from build123d import *

# Parameters (mm, degrees)
EXTRUDE_1_DEPTH     = 25
EXTRUDE_2_DEPTH     = 36
SKETCH_3_W          = 15
SKETCH_3_H          = 6
EXTRUDE_3_DEPTH     = 12
SKETCH_4_R          = 0.95
CUT_EXTRUDE_1_DEPTH = 21
SKETCH_5_R          = 4
SKETCH_5_R_2        = 1.45
EXTRUDE_4_DEPTH     = 20
EXTRUDE_4_2_DEPTH   = 20
SKETCH_6_R          = 1.75
CUT_EXTRUDE_2_DEPTH = 20
SKETCH_7_R          = 2.5
CUT_EXTRUDE_3_DEPTH = 2
CUT_EXTRUDE_4_DEPTH = 52.148040055
FILLET_4_R          = 1
SKETCH_9_W          = 2
SKETCH_9_H          = 14
EXTRUDE_5_DEPTH     = 20


with BuildPart() as part:
    # Sketch 1 → Extrude 1 (new, symmetric)
    with BuildSketch(Plane.XY):
        Polygon((0, 0), (9.650045346, 0), (39.194277936, -5.20944533), (39.888870647, -1.270214318), (10, 4), (0, 4), align=None)
    extrude_1 = extrude(amount=EXTRUDE_1_DEPTH, both=True)

    # Sketch 2 → Extrude 2 (add)
    with BuildSketch(Plane.XY.offset(25)):
        Polygon((22.162331093, 1.85545288), (22.483580221, 3.677347223), (37.255696517, 1.072624558), (36.934447388, -0.749269785), align=None)
    extrude_2 = extrude(amount=-EXTRUDE_2_DEPTH)

    # Sketch 3 → Extrude 3 (add)
    with BuildSketch(Plane(origin=(1.306826311, 7.411380301, 0), x_dir=(0.9848077530122079, -0.1736481776669312, 0), z_dir=(0.1736481776669312, 0.9848077530122079, 0))):
        with Locations((29.003439474, -22)):
            Rectangle(SKETCH_3_W, SKETCH_3_H)
        with Locations((29.003439474, 7.8)):
            Rectangle(SKETCH_3_W, SKETCH_3_H)
    extrude_3 = extrude(amount=EXTRUDE_3_DEPTH)

    # Sketch 4 → Cut-Extrude 1 (cut)
    with BuildSketch(Plane(origin=(35.948870205, -6.338755743, 0), x_dir=(0, 0, -1), z_dir=(0.9848077530122081, -0.17364817766693072, 0))):
        with Locations(Location((-20.95, 14.025712789, 0), (0, 0, 90))):
            Circle(SKETCH_4_R)
        with Locations(Location((6.75, 14.025712789, 0), (0, 0, 90))):
            Circle(SKETCH_4_R)
    cut_extrude_1 = extrude(amount=-CUT_EXTRUDE_1_DEPTH, mode=Mode.SUBTRACT)

    # Mirror 1: Extrude 1, Extrude 2, Extrude 3, Cut-Extrude 1 across plane
    add(extrude_1.mirror(Plane(origin=(0, 0, 0), x_dir=(0, 0, 1), z_dir=(1, 0, 0))))
    add(extrude_2.mirror(Plane(origin=(0, 0, 0), x_dir=(0, 0, 1), z_dir=(1, 0, 0))))
    add(extrude_3.mirror(Plane(origin=(0, 0, 0), x_dir=(0, 0, 1), z_dir=(1, 0, 0))))
    add(cut_extrude_1.mirror(Plane(origin=(0, 0, 0), x_dir=(0, 0, 1), z_dir=(1, 0, 0))), mode=Mode.SUBTRACT)

    # Sketch 6 → Cut-Extrude 2 (cut)
    with BuildSketch(Plane(origin=(0, 4, 0), x_dir=(1, 0, 0), z_dir=(0, 1, 0))):
        with Locations(Location((0, -20, 0), (0, 0, 180))):
            Circle(SKETCH_6_R)
        with Locations((-13, 9.5)):
            Circle(SKETCH_6_R)
        with Locations(Location((13, 9.5, 0), (0, 0, 180))):
            Circle(SKETCH_6_R)
    extrude(amount=-CUT_EXTRUDE_2_DEPTH, mode=Mode.SUBTRACT)

    # Sketch 7 → Cut-Extrude 3 (cut)
    with BuildSketch(Plane(origin=(0, 4, 0), x_dir=(1, 0, 0), z_dir=(0, 1, 0))):
        with Locations(Location((-13, 9.5, 0), (0, 0, 180))):
            Circle(SKETCH_7_R)
        with Locations(Location((13, 9.5, 0), (0, 0, 180))):
            Circle(SKETCH_7_R)
    extrude(amount=-CUT_EXTRUDE_3_DEPTH, mode=Mode.SUBTRACT)

    # Sketch 8 → Cut-Extrude 4 (cut, through all)
    with BuildSketch(Plane(origin=(0, 4, 0), x_dir=(1, 0, 0), z_dir=(0, 1, 0))):
        Polygon((-4, 23), (-1, 23), (-1, 25), (1, 25), (1, 23), (4, 23), (4, 14), (-4, 14), align=None)
    extrude(amount=-CUT_EXTRUDE_4_DEPTH, mode=Mode.SUBTRACT)

    # Fillet 4
    fillet_4_edges = [part.edges().sort_by_distance(p)[0] for p in [
        (4, 2, -23),
        (4, 2, -14),
        (-4, 2, -14),
        (-4, 2, -23),
        (1, 2, -23),
        (-1, 2, -23),
    ]]
    fillet(fillet_4_edges, radius=FILLET_4_R)



with BuildPart() as body_2:
    # Sketch 5 → Extrude 4 (new body)
    with BuildSketch(Plane(origin=(0, 4, 0), x_dir=(1, 0, 0), z_dir=(0, 1, 0))):
        with Locations(Location((0, -12, 0), (0, 0, 180))):
            Circle(SKETCH_5_R)
        with Locations(Location((0, -12, 0), (0, 0, 180))):
            Circle(SKETCH_5_R_2, mode=Mode.SUBTRACT)
    extrude(amount=EXTRUDE_4_DEPTH)


with BuildPart() as body_3:
    # Sketch 5 → Extrude 4 2 (new body)
    with BuildSketch(Plane(origin=(0, 4, 0), x_dir=(1, 0, 0), z_dir=(0, 1, 0))):
        with Locations(Location((0, 8, 0), (0, 0, 180))):
            Circle(SKETCH_5_R)
        with Locations(Location((0, 8, 0), (0, 0, 180))):
            Circle(SKETCH_5_R_2, mode=Mode.SUBTRACT)
    extrude(amount=EXTRUDE_4_2_DEPTH)


with BuildPart() as part_1:
    add(part.part)

    add(body_2.part)  # Extrude 5 merges body 2

    add(body_3.part)  # Extrude 5 merges body 3
    # Sketch 9 → Extrude 5 (add)
    with BuildSketch(Plane(origin=(0, 4, 0), x_dir=(1, 0, 0), z_dir=(0, 1, 0))):
        with Locations((0, -2)):
            Rectangle(SKETCH_9_W, SKETCH_9_H)
    extrude(amount=EXTRUDE_5_DEPTH)


solid = part_1.part
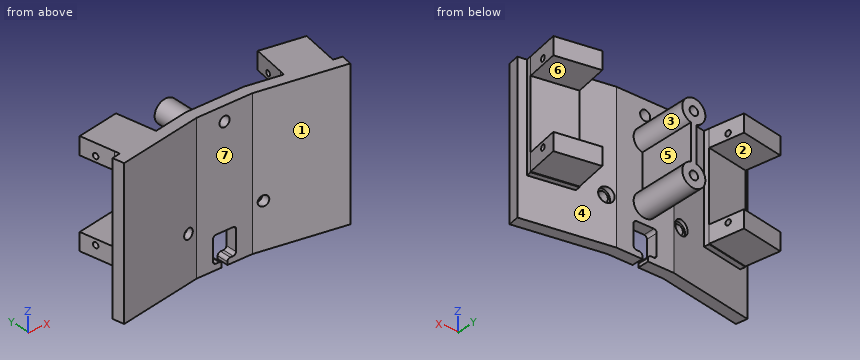
Here's how the part is built. I have some questions about the finished solid (model axes, mm). Face numbers are marked on the shaded views. A direction names the side the tool comes from. Round coordinates to 2 decimals unless told otherwise and drop trailing zeros. Order: outer loops, then holes, each group sorted by start corner. A loop starts at its lowest first (then second) coordinate and runs counter-clockwise, first axis right, second up. Notation, with made-up numbers: M 27.5,78.25 L 53.5,78.25 A36 cw 53.5,112.25 Z; hole C 47,48.5 d1. An arc over 180 degrees is marked long. Return JSON: item names as keys, results as strings. Group by question number.
1. If we section it at A-A on x = 0: List the corners of the cut face in (y, z) for me, then the cut area to 3 significant figures.
2. If we section it at D-D on x = -13: List the corners of the cut face in (y, z) for me, then the cut area to 3 significant figures.
3. If we section it at B-B on z = 12: List the corners of the cut face in (x, y) for me.
4. If we mould it in two halves opening along X, with no side actions, what happens to the marked faces 4, 5, 6 and 7? For each: pulls with the +X half, pulls with the -X half, needs draft (parallel to the pull), parting line crosses it, or undercut.
5. On a 3-axis mill with a long thin cutter (end or side, diameter ignored), from which of +Z, -Z, +X, -X, +Y, -Y can I reach the whole of each face in a straight line? I mean the marked faces 1, 2 and 3. Say none if no direction works.
6. Please list where these lines run through material, in increasing order: probe 1 along Z at (x, y) = (13, 0); probe 2 along Z at (x, y) = (0, 11.5); probe 3 along Z at (x, y) = (-33, 4.25).
7. I'm going to push flat-ended pins straight in: pin 1 Ø7 at (x, y) = (28, 10) entering from -Z; pin 2 Ø6 at (x, z) = (9, -13.5) entering from +Y; pin 3 Ø6 at (x, z) = (18.5, 2) entering from +Y. Where does each tip first touch, or does it pass through?
8. If we section it at C-C on x = -30.5: State how many separate pieces and enclosed holes the cut face has, then the cut area to 3 significant figures.
Reply:
{
 "1": {"outline": "M 0,-14 L 4,-14 L 4,-12 L 24,-12 L 24,-9.45 L 4,-9.45 L 4,-6.55 L 24,-6.55 L 24,10.55 L 4,10.55 L 4,13.45 L 24,13.45 L 24,16 L 4,16 L 4,18.25 L 0,18.25 Z; M 0,21.75 L 4,21.75 L 4,25 L 0,25 Z", "area": "586 mm^2"},
 "2": {"outline": "M -0.59,-25 L 3.47,-25 L 3.47,-12 L 2,-12 L 2,-11.25 L -0.59,-11.25 Z; M -0.59,-7.75 L 2,-7.75 L 2,-7 L 3.47,-7 L 3.47,25 L -0.59,25 Z", "area": "187 mm^2"},
 "3": {"outline": "M -39.89,-1.27 L -39.19,-5.21 L -9.65,0 L 9.65,0 L 39.19,-5.21 L 39.89,-1.27 L 36.93,-0.75 L 37.26,1.07 L 22.48,3.68 L 22.16,1.86 L 10,4 L 4,4 L 4,24 L 1.45,24 L 1.45,4 L -1.45,4 L -1.45,24 L -4,24 L -4,4 L -10,4 L -22.16,1.86 L -22.48,3.68 L -37.26,1.07 L -36.93,-0.75 Z"},
 "4": {"face 4": "undercut", "face 5": "pulls with the +X half", "face 6": "needs draft", "face 7": "undercut"},
 "5": {"face 1": "+Z, -Z, -Y", "face 2": "-X, +Y", "face 3": "+Y"},
 "6": {"probe 1": "-25 to -11.25, -7.75 to 25", "probe 2": "-12 to -9.45, -6.55 to 10.55, 13.45 to 16", "probe 3": "-10.8 to -4.8, 19 to 25"},
 "7": {"pin 1": "z = -10.8", "pin 2": "y = 4", "pin 3": "y = 3.03"},
 "8": {"separate pieces": "1", "enclosed holes": "2", "area": "411 mm^2"}
}
